Source: CAD feature listing. Evaluate the final solid. Frame: model axes, mm. Give positions to 0.01 mm unless a question says otherwise; leave off trailing zeros. Write each loop counter-clockwise with the first axis right and the second up, starting at its lowest first coordinate (ties: lowest second). Pieces come first, ordered by that corner, then holes. Notation, with made-up numbers: (38, 74.5) -> (46, 74.5) arc R21 ccw to (46, 86.5) -> close; hole circle Ø3 at (-2, 49). An arc over 180 degrees is marked (long way). Answer as a JSON object with one key per item and string values. Group by question number.
Item 1: Section query A-A on y = 0. Return the cut outline in (x, z).
Item 2: First-contact query: pin 1 Ø6.5 at (x, y) = (45, 0) entering from -Z; pin 2 Ø1 at (x, z) = (20.5, 1) entering from +Y; pin 3 Ø3 at (x, z) = (-16, 4) entering from +Y. Flat tips, straight axial feed; report the tip coordinate or a pass-through.
Item 3: Section query B-B on z = 1.95. Return the cut outline in (x, y).
Item 4: Ray query, probe 1 along X at (y, z) = (-0.5, 1.3); probe 2 along Y at (x, z) = (-45, 0.95); probe 3 along Y at (x, z) = (33, 1.1). Return the intervals inside material, ascending. Write a range as from..to.
Item 5: Pull-direction query (Y, two-part tool) for faces 1 (the face through (42, 0, 4)), 2 (the face through (49.738, 15.663, 5.854)), 3 (the face through (-1, 1, 0)); classes: pulls with the +Y half, pulls with the -Y half, needs draft (parallel to the pull), parting line crosses it, or undercut.
from build123d import *

# Parameters (mm, degrees)
F0_R     = 55
F0_R_2   = 2.5
F1_DEPTH = 6
F2_SIZE  = 3
F3_SIZE  = 2.5


with BuildPart() as f1:
    # F0 (on Top) → F1 (new body)
    with BuildSketch(Plane.XY):
        Circle(F0_R)
        with Locations((-45, 0)):
            Circle(F0_R_2, mode=Mode.SUBTRACT)
        with Locations((45, 0)):
            Circle(F0_R_2, mode=Mode.SUBTRACT)
    extrude(amount=F1_DEPTH)

    # F2
    f2_edges = [f1.edges().sort_by_distance(p)[0] for p in [
        (-55, 0, 6),
    ]]
    chamfer(f2_edges, length=F2_SIZE)

    # F3
    f3_edges = [f1.edges().sort_by_distance(p)[0] for p in [
        (-47.5, 0, 6),
        (42.5, 0, 6),
    ]]
    chamfer(f3_edges, length=F3_SIZE)


solid = f1.part
Worked answers:
{
 "1": {"outline": "(-55, 0) -> (-47.5, 0) -> (-47.5, 3.5) -> (-50, 6) -> (-52, 6) -> (-55, 3) -> close; (-42.5, 0) -> (42.5, 0) -> (42.5, 3.5) -> (40, 6) -> (-40, 6) -> (-42.5, 3.5) -> close; (47.5, 0) -> (55, 0) -> (55, 3) -> (52, 6) -> (50, 6) -> (47.5, 3.5) -> close"},
 "2": {"pin 1": "z = 0", "pin 2": "y = 51.23", "pin 3": "y = 52.95"},
 "3": {"outline": "circle Ø110 at (0, 0); hole circle Ø5 at (-45, 0); hole circle Ø5 at (45, 0)"},
 "4": {"probe 1": "-55..-47.45, -42.55..42.55, 47.45..55", "probe 2": "-31.62..-2.5, 2.5..31.62", "probe 3": "-44..44"},
 "5": {"face 1": "undercut", "face 2": "parting line crosses it", "face 3": "needs draft"}
}
